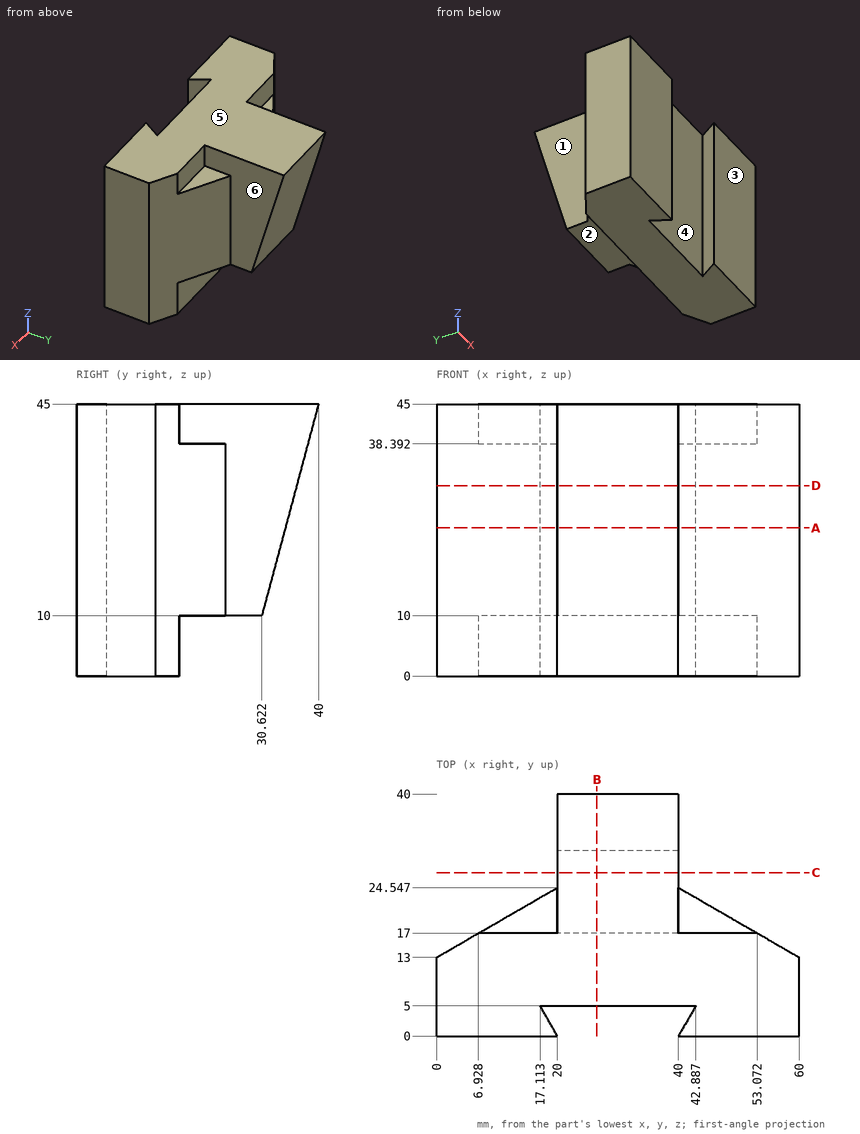
Check sheet for the drawn part. Datum: minimum x, y, z corner. Units: mm. A direction names the side the tool comes from. Coordinates: 2 decimals unless noted, no trailing zeros. Order: outer loops, then holes, each group sorted by start corner. A loop starts at its lowest first (then second) coordinate and runs counter-clockwise, first axis right, second up. Notation, with made-up numbers: (40.5, -27) -> (96.5, -27) arc R17 cw to (96.5, 3) -> close; hole circle Ø7 at (24, 33). An arc over 180 degrees is marked (long way). Use a Markdown table: item, result. Add a question column.
1. Material ranges on L1, parallel to Y at x = 39.5, z = 39; L2, parallel to Y at x = 51.5, z = 39; L3, parallel to X at y = 29, z = 43.5, recorded low to high.
2. Cross-section at A-A (z = 24.5). Enter the section's corners in (x, y), and give its area (3 significant figures).
3. Set-up check for the marked faces 1, 2 and 3: record each of +Z, -Z, +X, -X, +Y, -Y from which the full face is reachable in a straight line by a thin tool's end or side.
4. Cross-section at B-B (x = 26.5). Enter the section's corners in (y, z).
5. Go/stop test with flat-tipped pins: pin 1 Ø12 at (x, y) = (33.5, 30) entering from -Z; pin 2 Ø11.5 at (y, z) = (28, 30) entering from -X; pin 3 Ø8 at (x, z) = (20, 26) entering from +Y. Record where each tip stops, or that it passes through.
6. Cross-section at C-C (y = 27). Enter the section's corners in (x, z).
7. Mould release check, pull along X, two halves, no side actions. Record for the marked faces 4, 5 and 6: pulls with the +X half, pulls with the -X half, needs draft (parallel to the pull), parting line crosses it, or undercut.
8. Cross-section at D-D (z = 31.5). Enter the section's corners in (x, y).
Filled sheet:
| question | item | result |
|---|---|---|
| 1 | L1 | 5 to 38.39 |
| 1 | L2 | 0 to 17 |
| 1 | L3 | 20 to 40 |
| 2 | outline | (0, 0) -> (20, 0) -> (17.11, 5) -> (42.89, 5) -> (40, 0) -> (60, 0) -> (60, 13) -> (40, 24.55) -> (40, 34.51) -> (20, 34.51) -> (20, 24.55) -> (0, 13) -> close |
| 2 | area | 1,330 mm2 |
| 3 | face 1 | +Z, -X, +Y |
| 3 | face 2 | -Z, +X, -X, +Y |
| 3 | face 3 | +Z, -Z, +X, -X, -Y |
| 4 | outline | (5, 0) -> (17, 0) -> (17, 10) -> (30.62, 10) -> (40, 45) -> (5, 45) -> close |
| 5 | pin 1 | z = 10 |
| 5 | pin 2 | x = 16.02 |
| 5 | pin 3 | y = 35.98 |
| 6 | outline | (20, 10) -> (40, 10) -> (40, 45) -> (20, 45) -> close |
| 7 | face 4 | undercut |
| 7 | face 5 | needs draft |
| 7 | face 6 | pulls with the +X half |
| 8 | outline | (0, 0) -> (20, 0) -> (17.11, 5) -> (42.89, 5) -> (40, 0) -> (60, 0) -> (60, 13) -> (40, 24.55) -> (40, 36.38) -> (20, 36.38) -> (20, 24.55) -> (0, 13) -> close |
